Part print with two shaded views. Sizes in mm from the minimum x, y, z corner. A direction names the side the tool comes from. Coordinates: 2 decimals unless noted, no trailing zeros. Loops run counter-clockwise (first coordinate to the right, second up) from the corner with the lowest first, then second, coordinate; pieces in that order, holes last. Notation, with made-up numbers: M -17.5,84 L 24.5,84 A9 ccw 24.5,89 Z; hole C 64,-12.5 d2. An arc over 180 degrees is marked long. Use CSV: the item, a comma, the result in double quotes. Start each with the question number.
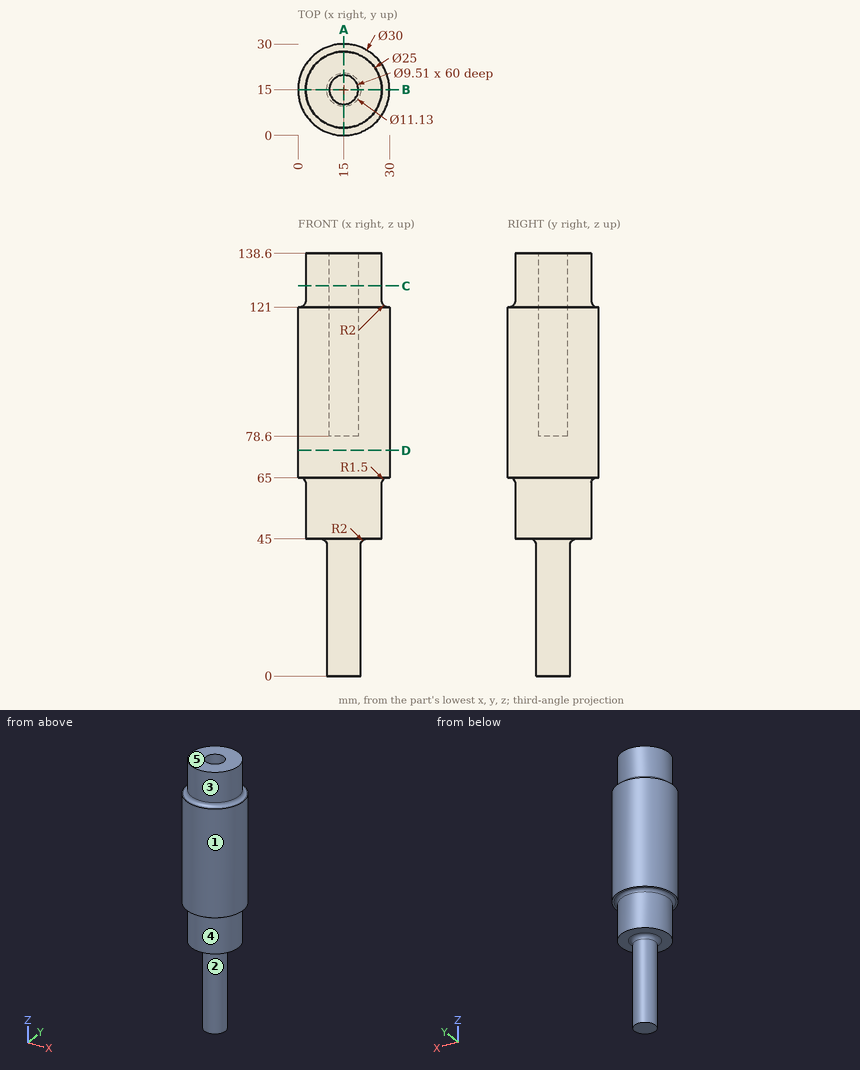
1. Slice it at D-D, the plane z = 74. List the corners of the cut face in (x, y).
2. Slice it at A-A, the plane x = 15. List the corners of the cut face in (y, z) (3 decimals).
3. Pin check, flat tips, straight feed: pin 1 (12 mm diameter, centred on x = 22.5, z = 93.5, fed in from +Y); pin 2 (1.5 mm diameter, centred on x = 20, z = 82.5, fed in from +Y); pin 3 (4 mm diameter, centred on y = 12.5, z = 73.5, fed in from +X); pin 4 (2 mm diameter, centred on x = 7.5, z = 38.5, fed in from +Y). Stop position of each tip, or through.
4. Slice it at C-C, the plane z = 128. List the corners of the cut face in (x, y) (3 decimals), and give its area (3 significant figures).
5. Two-plate mould, pull along Z, no slides. Class the marked faces 4 and 5: pulls with the +Z half, pulls with the -Z half, needs draft (parallel to the pull), parting line crosses it, or undercut.
6. Tool access for the marked faces 1, 2 and 3: list every direction of +Z, -Z, +X, -X, +Y, -Y with a clear straight run to the whole face (end or side of a thin tool).
7. Wall check: probe 1 along Y at (x, z) = (15, 98.5) (3 decimals); probe 2 along Z at (x, y) = (15, 26); probe 3 along Y at (x, z) = (12, 128). Give the ranges that are in metal, low to high.
Found:
1,outline,"C 15,15 d30"
2,outline,"M 0,65 L 1,65 A1.5 cw 2.5,63.5 L 2.5,45 L 7.435,45 A2 cw 9.435,43 L 9.435,0 L 20.565,0 L 20.565,43 A2 cw 22.565,45 L 27.5,45 L 27.5,63.5 A1.5 cw 29,65 L 30,65 L 30,121 L 29.5,121 A2 cw 27.5,123 L 27.5,138.6 L 19.755,138.6 L 19.755,78.6 L 10.245,78.6 L 10.245,138.6 L 2.5,138.6 L 2.5,123 A2 cw 0.5,121 L 0,121 Z"
3,pin 1,"y = 29.92"
3,pin 2,"y = 29.39"
3,pin 3,"x = 29.99"
3,pin 4,"through"
4,outline,"C 15,15 d25; hole C 15,15 d9.51"
4,area,"420 mm^2"
5,face 4,"needs draft"
5,face 5,"pulls with the +Z half"
6,face 1,"+Z, -Z"
6,face 2,"-Z"
6,face 3,"+Z"
7,probe 1,"0 to 10.245, 19.755 to 30"
7,probe 2,"45 to 138.6"
7,probe 3,"2.87 to 11.31, 18.69 to 27.13"
